from build123d import *

# Parameters (mm, degrees)
SKETCH1_W               = 3.175
SKETCH1_H               = 19.05
CUT_EXTRUDE2_DEPTH      = 11.530283709
CUT_EXTRUDE2_DEPTH_BACK = 11.530283709
SKETCH3_W               = 0.396875
SKETCH3_H               = 6.35
FILLET3_R               = 0.1984375
CHAMFER1_SIZE           = 0.762


with BuildPart() as part:
    # Sketch1 → Revolve1 (revolve)
    with BuildSketch(Plane.XY, mode=Mode.PRIVATE) as revolve1_sk:
        with Locations((1.5875, 0)):
            Rectangle(SKETCH1_W, SKETCH1_H)
    revolve(revolve1_sk.sketch.rotate(Axis((0, 5.054239483, 0), (0, -1, 0)), 90), axis=Axis((0, 5.054239483, 0), (0, -1, 0)))

    # Sketch3 → Cut-Extrude2 (cut, two sides: drawn at the far end of the back side and taken through both)
    with BuildSketch(Plane.XY.offset(-CUT_EXTRUDE2_DEPTH_BACK)):
        with Locations((2.9765625, 0)):
            Rectangle(SKETCH3_W, SKETCH3_H)
    extrude(amount=CUT_EXTRUDE2_DEPTH + CUT_EXTRUDE2_DEPTH_BACK, mode=Mode.SUBTRACT)

    # Fillet3
    fillet3_edges = [part.edges().sort_by_distance(p)[0] for p in [
        (2.778125, -3.175, 0),
        (2.778125, 3.175, 0),
    ]]
    fillet(fillet3_edges, radius=FILLET3_R)
    fillet3_2_edges = [part.edges().sort_by_distance(p)[0] for p in [
        (2.778125, 0, 1.537090266),
        (2.778125, 0, -1.537090266),
        (2.842710111, 3.123058164, -1.414080692),
        (2.842706566, -3.123054925, -1.41408782),
        (2.842710111, 3.123058164, 1.414080692),
        (2.842706566, -3.123054925, 1.41408782),
    ]]
    fillet(fillet3_2_edges, radius=FILLET3_R - 0.0001)  # a hair under: the kernel refuses the full size

    # Chamfer1
    chamfer1_edges = [part.edges().sort_by_distance(p)[0] for p in [
        (0, -9.525, -3.175),
        (0, 9.525, -3.175),
    ]]
    chamfer(chamfer1_edges, length=CHAMFER1_SIZE)


solid = part.part
Verification items for the finished model (mm, model axes). Coordinates: 2 decimals unless noted, no trailing zeros. Order: outer loops, then holes, each group sorted by start corner. A loop starts at its lowest first (then second) coordinate and runs counter-clockwise, first axis right, second up. Notation, with made-up numbers: M 57,22 L 92,22 A17 cw 92,43 Z; hole C 72,78.25 d9. An arc over 180 degrees is marked long. One line per item, written item: value. Start each with the question number.
Item 1: Sectioned sample at B-B (y = -8). Enter the section's corners in (x, z) (3 decimals), then the cut area to 3 significant figures.
Item 2: Mould release check, pull along Y, two halves, no side actions. Record for faces 1 (the flat face through (2.778, 0, 0)), 2 (the cylindrical face through (-3.15, 0.12, -0.41)), 3 (the flat face through (0, 9.525, 0)): released by +Y, released by -Y, zero draft, split by the parting line, or undercut.
Item 3: Sectioned sample at A-A (y = -0.25). Enter the section's corners in (x, z) (3 decimals).
Item 4: Scan lines: probe 1 along X at (y, z) = (-5.75, 2.5); probe 2 along Z at (x, y) = (1.5, 8.5); probe 3 along Z at (x, y) = (0.5, 1.5). Record each from-to range of solid material in increasing order.
Item 5: Gauge pin test, flat ends, axial feed: pin 1 (2 mm diameter, centred on y = -3, z = -1.5, fed in from +X); pin 2 (2 mm diameter, centred on y = -5.5, z = -2, fed in from +X); pin 3 (2.5 mm diameter, centred on y = 0, z = -0.5, fed in from +X). Record the tip position at first contact, or that the pin passes through.
Conclusion:
1. outline: C 0,0 d6.35
1. area: 31.7 mm^2
2. face 1: undercut
2. face 2: zero draft
2. face 3: released by +Y
3. outline: M 2.752,-1.584 A0.198 ccw 2.778,-1.485 L 2.778,1.485 A0.198 ccw 2.752,1.584 A3.175 ccw long Z
4. probe 1: x = -1.96 to 1.96
4. probe 2: z = -2.8 to 2.8
4. probe 3: z = -3.14 to 3.14
5. pin 1: stops at x = 3.12
5. pin 2: stops at x = 3.01
5. pin 3: stops at x = 2.78
